```python
from build123d import *

# Parameters (mm, degrees)
SKETCH_2_R      = 300
SKETCH_2_R_2    = 3
EXTRUDE_1_DEPTH = 20


with BuildPart() as part:
    # Эскиз2 → Бобышка-Вытянуть1 (new body)
    with BuildSketch(Plane(origin=(0, 0, 0), x_dir=(1, 0, 0), z_dir=(0, 1, 0))):
        with Locations(Location((0, 0, 0), (0, 0, 270))):
            Circle(SKETCH_2_R)
        with Locations(Location((-50, 50, 0), (0, 0, 270))):
            Circle(SKETCH_2_R_2, mode=Mode.SUBTRACT)
        with Locations(Location((-100, 50, 0), (0, 0, 270))):
            Circle(SKETCH_2_R_2, mode=Mode.SUBTRACT)
        with Locations(Location((-150, 50, 0), (0, 0, 270))):
            Circle(SKETCH_2_R_2, mode=Mode.SUBTRACT)
        with Locations(Location((-200, 50, 0), (0, 0, 270))):
            Circle(SKETCH_2_R_2, mode=Mode.SUBTRACT)
        with Locations(Location((-50, 100, 0), (0, 0, 270))):
            Circle(SKETCH_2_R_2, mode=Mode.SUBTRACT)
        with Locations(Location((-100, 100, 0), (0, 0, 270))):
            Circle(SKETCH_2_R_2, mode=Mode.SUBTRACT)
        with Locations(Location((-150, 100, 0), (0, 0, 270))):
            Circle(SKETCH_2_R_2, mode=Mode.SUBTRACT)
        with Locations(Location((-200, 100, 0), (0, 0, 270))):
            Circle(SKETCH_2_R_2, mode=Mode.SUBTRACT)
        with Locations(Location((-250, 100, 0), (0, 0, 270))):
            Circle(SKETCH_2_R_2, mode=Mode.SUBTRACT)
        with Locations(Location((-50, 150, 0), (0, 0, 270))):
            Circle(SKETCH_2_R_2, mode=Mode.SUBTRACT)
        with Locations(Location((-100, 150, 0), (0, 0, 270))):
            Circle(SKETCH_2_R_2, mode=Mode.SUBTRACT)
        with Locations(Location((-150, 150, 0), (0, 0, 270))):
            Circle(SKETCH_2_R_2, mode=Mode.SUBTRACT)
        with Locations(Location((-200, 150, 0), (0, 0, 270))):
            Circle(SKETCH_2_R_2, mode=Mode.SUBTRACT)
        with Locations(Location((-50, 200, 0), (0, 0, 270))):
            Circle(SKETCH_2_R_2, mode=Mode.SUBTRACT)
        with Locations(Location((-100, 200, 0), (0, 0, 270))):
            Circle(SKETCH_2_R_2, mode=Mode.SUBTRACT)
        with Locations(Location((-150, 200, 0), (0, 0, 270))):
            Circle(SKETCH_2_R_2, mode=Mode.SUBTRACT)
        with Locations(Location((-100, 250, 0), (0, 0, 270))):
            Circle(SKETCH_2_R_2, mode=Mode.SUBTRACT)
        with Locations(Location((-50, 0, 0), (0, 0, 270))):
            Circle(SKETCH_2_R_2, mode=Mode.SUBTRACT)
        with Locations(Location((-150, 0, 0), (0, 0, 270))):
            Circle(SKETCH_2_R_2, mode=Mode.SUBTRACT)
        with Locations(Location((-100, 0, 0), (0, 0, 270))):
            Circle(SKETCH_2_R_2, mode=Mode.SUBTRACT)
        with Locations(Location((-200, 0, 0), (0, 0, 270))):
            Circle(SKETCH_2_R_2, mode=Mode.SUBTRACT)
        with Locations(Location((0, 50, 0), (0, 0, 270))):
            Circle(SKETCH_2_R_2, mode=Mode.SUBTRACT)
        with Locations(Location((0, 100, 0), (0, 0, 270))):
            Circle(SKETCH_2_R_2, mode=Mode.SUBTRACT)
        with Locations(Location((0, 150, 0), (0, 0, 270))):
            Circle(SKETCH_2_R_2, mode=Mode.SUBTRACT)
        with Locations(Location((0, 200, 0), (0, 0, 270))):
            Circle(SKETCH_2_R_2, mode=Mode.SUBTRACT)
        with Locations(Location((200, 0, 0), (0, 0, 90))):
            Circle(SKETCH_2_R_2, mode=Mode.SUBTRACT)
        with Locations(Location((100, 0, 0), (0, 0, 90))):
            Circle(SKETCH_2_R_2, mode=Mode.SUBTRACT)
        with Locations(Location((150, 0, 0), (0, 0, 90))):
            Circle(SKETCH_2_R_2, mode=Mode.SUBTRACT)
        with Locations(Location((50, 0, 0), (0, 0, 90))):
            Circle(SKETCH_2_R_2, mode=Mode.SUBTRACT)
        with Locations(Location((100, 250, 0), (0, 0, 90))):
            Circle(SKETCH_2_R_2, mode=Mode.SUBTRACT)
        with Locations(Location((150, 200, 0), (0, 0, 90))):
            Circle(SKETCH_2_R_2, mode=Mode.SUBTRACT)
        with Locations(Location((100, 200, 0), (0, 0, 90))):
            Circle(SKETCH_2_R_2, mode=Mode.SUBTRACT)
        with Locations(Location((50, 200, 0), (0, 0, 90))):
            Circle(SKETCH_2_R_2, mode=Mode.SUBTRACT)
        with Locations(Location((200, 150, 0), (0, 0, 90))):
            Circle(SKETCH_2_R_2, mode=Mode.SUBTRACT)
        with Locations(Location((150, 150, 0), (0, 0, 90))):
            Circle(SKETCH_2_R_2, mode=Mode.SUBTRACT)
        with Locations(Location((100, 150, 0), (0, 0, 90))):
            Circle(SKETCH_2_R_2, mode=Mode.SUBTRACT)
        with Locations(Location((50, 150, 0), (0, 0, 90))):
            Circle(SKETCH_2_R_2, mode=Mode.SUBTRACT)
        with Locations(Location((250, 100, 0), (0, 0, 90))):
            Circle(SKETCH_2_R_2, mode=Mode.SUBTRACT)
        with Locations(Location((200, 100, 0), (0, 0, 90))):
            Circle(SKETCH_2_R_2, mode=Mode.SUBTRACT)
        with Locations(Location((150, 100, 0), (0, 0, 90))):
            Circle(SKETCH_2_R_2, mode=Mode.SUBTRACT)
        with Locations(Location((100, 100, 0), (0, 0, 90))):
            Circle(SKETCH_2_R_2, mode=Mode.SUBTRACT)
        with Locations(Location((50, 100, 0), (0, 0, 90))):
            Circle(SKETCH_2_R_2, mode=Mode.SUBTRACT)
        with Locations(Location((200, 50, 0), (0, 0, 90))):
            Circle(SKETCH_2_R_2, mode=Mode.SUBTRACT)
        with Locations(Location((150, 50, 0), (0, 0, 90))):
            Circle(SKETCH_2_R_2, mode=Mode.SUBTRACT)
        with Locations(Location((100, 50, 0), (0, 0, 90))):
            Circle(SKETCH_2_R_2, mode=Mode.SUBTRACT)
        with Locations(Location((50, 50, 0), (0, 0, 90))):
            Circle(SKETCH_2_R_2, mode=Mode.SUBTRACT)
        with Locations(Location((50, -50, 0), (0, 0, 270))):
            Circle(SKETCH_2_R_2, mode=Mode.SUBTRACT)
        with Locations(Location((100, -50, 0), (0, 0, 270))):
            Circle(SKETCH_2_R_2, mode=Mode.SUBTRACT)
        with Locations(Location((150, -50, 0), (0, 0, 270))):
            Circle(SKETCH_2_R_2, mode=Mode.SUBTRACT)
        with Locations(Location((200, -50, 0), (0, 0, 270))):
            Circle(SKETCH_2_R_2, mode=Mode.SUBTRACT)
        with Locations(Location((50, -100, 0), (0, 0, 270))):
            Circle(SKETCH_2_R_2, mode=Mode.SUBTRACT)
        with Locations(Location((100, -100, 0), (0, 0, 270))):
            Circle(SKETCH_2_R_2, mode=Mode.SUBTRACT)
        with Locations(Location((150, -100, 0), (0, 0, 270))):
            Circle(SKETCH_2_R_2, mode=Mode.SUBTRACT)
        with Locations(Location((200, -100, 0), (0, 0, 270))):
            Circle(SKETCH_2_R_2, mode=Mode.SUBTRACT)
        with Locations(Location((250, -100, 0), (0, 0, 270))):
            Circle(SKETCH_2_R_2, mode=Mode.SUBTRACT)
        with Locations(Location((50, -150, 0), (0, 0, 270))):
            Circle(SKETCH_2_R_2, mode=Mode.SUBTRACT)
        with Locations(Location((100, -150, 0), (0, 0, 270))):
            Circle(SKETCH_2_R_2, mode=Mode.SUBTRACT)
        with Locations(Location((150, -150, 0), (0, 0, 270))):
            Circle(SKETCH_2_R_2, mode=Mode.SUBTRACT)
        with Locations(Location((200, -150, 0), (0, 0, 270))):
            Circle(SKETCH_2_R_2, mode=Mode.SUBTRACT)
        with Locations(Location((50, -200, 0), (0, 0, 270))):
            Circle(SKETCH_2_R_2, mode=Mode.SUBTRACT)
        with Locations(Location((100, -200, 0), (0, 0, 270))):
            Circle(SKETCH_2_R_2, mode=Mode.SUBTRACT)
        with Locations(Location((150, -200, 0), (0, 0, 270))):
            Circle(SKETCH_2_R_2, mode=Mode.SUBTRACT)
        with Locations(Location((100, -250, 0), (0, 0, 270))):
            Circle(SKETCH_2_R_2, mode=Mode.SUBTRACT)
        with Locations(Location((0, -200, 0), (0, 0, 90))):
            Circle(SKETCH_2_R_2, mode=Mode.SUBTRACT)
        with Locations(Location((0, -150, 0), (0, 0, 90))):
            Circle(SKETCH_2_R_2, mode=Mode.SUBTRACT)
        with Locations(Location((0, -100, 0), (0, 0, 90))):
            Circle(SKETCH_2_R_2, mode=Mode.SUBTRACT)
        with Locations(Location((0, -50, 0), (0, 0, 90))):
            Circle(SKETCH_2_R_2, mode=Mode.SUBTRACT)
        with Locations(Location((-100, -250, 0), (0, 0, 90))):
            Circle(SKETCH_2_R_2, mode=Mode.SUBTRACT)
        with Locations(Location((-150, -200, 0), (0, 0, 90))):
            Circle(SKETCH_2_R_2, mode=Mode.SUBTRACT)
        with Locations(Location((-100, -200, 0), (0, 0, 90))):
            Circle(SKETCH_2_R_2, mode=Mode.SUBTRACT)
        with Locations(Location((-50, -200, 0), (0, 0, 90))):
            Circle(SKETCH_2_R_2, mode=Mode.SUBTRACT)
        with Locations(Location((-200, -150, 0), (0, 0, 90))):
            Circle(SKETCH_2_R_2, mode=Mode.SUBTRACT)
        with Locations(Location((-150, -150, 0), (0, 0, 90))):
            Circle(SKETCH_2_R_2, mode=Mode.SUBTRACT)
        with Locations(Location((-100, -150, 0), (0, 0, 90))):
            Circle(SKETCH_2_R_2, mode=Mode.SUBTRACT)
        with Locations(Location((-50, -150, 0), (0, 0, 90))):
            Circle(SKETCH_2_R_2, mode=Mode.SUBTRACT)
        with Locations(Location((-250, -100, 0), (0, 0, 90))):
            Circle(SKETCH_2_R_2, mode=Mode.SUBTRACT)
        with Locations(Location((-200, -100, 0), (0, 0, 90))):
            Circle(SKETCH_2_R_2, mode=Mode.SUBTRACT)
        with Locations(Location((-150, -100, 0), (0, 0, 90))):
            Circle(SKETCH_2_R_2, mode=Mode.SUBTRACT)
        with Locations(Location((-100, -100, 0), (0, 0, 90))):
            Circle(SKETCH_2_R_2, mode=Mode.SUBTRACT)
        with Locations(Location((-50, -100, 0), (0, 0, 90))):
            Circle(SKETCH_2_R_2, mode=Mode.SUBTRACT)
        with Locations(Location((-200, -50, 0), (0, 0, 90))):
            Circle(SKETCH_2_R_2, mode=Mode.SUBTRACT)
        with Locations(Location((-150, -50, 0), (0, 0, 90))):
            Circle(SKETCH_2_R_2, mode=Mode.SUBTRACT)
        with Locations(Location((-100, -50, 0), (0, 0, 90))):
            Circle(SKETCH_2_R_2, mode=Mode.SUBTRACT)
        with Locations(Location((-50, -50, 0), (0, 0, 90))):
            Circle(SKETCH_2_R_2, mode=Mode.SUBTRACT)
    extrude(amount=EXTRUDE_1_DEPTH)


solid = part.part
```
Part model, mm, in its own coordinate system. Round coordinates to 2 decimals unless told otherwise and drop trailing zeros. Write each loop counter-clockwise with the first axis right and the second up, starting at its lowest first coordinate (ties: lowest second). Pieces come first, ordered by that corner, then holes. Notation, with made-up numbers: M -12,-2 L 25,-2 A21 cw 25,33 Z; hole C 3.25,22.25 d10. An arc over 180 degrees is marked long. One line per question, with ' | ' between items.
(1) Saw through at A-A on y = 13. Count the separate pieces of the cut face and the enclosed holes in it, then the cut area to 3 significant figures.
Answer key:
separate pieces: 1 | enclosed holes: 84 | area: 280,000 mm^2
(2) Probe line 1 along X through (y, z) = (15.25, 260.5); line 2 along X through (y, z) = (3, -155); line 3 along Z through (x, y) = (132, 15.25). List the from-to ranges inside material, lowest first.
Answer key:
line 1: x = -148.79 to 148.79 | line 2: x = -256.86 to 256.86 | line 3: z = -269.4 to 269.4
(3) Pin check, flat tips, straight feed: pin 1 (2 mm diameter, centred on x = -106, y = 14.5, fed in from -Z); pin 2 (12 mm diameter, centred on y = 12, z = -97, fed in from -X); pin 3 (8 mm diameter, centred on x = 108.5, y = 16, fed in from +Z). Stop position of each tip, or through.
Answer key:
pin 1: stops at z = -281.02 | pin 2: stops at x = -285.87 | pin 3: stops at z = 281.21
(4) Saw through at C-C on z = 135. Write the cut outline in (x, y).
Answer key:
outline: M -267.91,0 L 267.91,0 L 267.91,20 L -267.91,20 Z
(5) Saw through at B-B on x = -76. Write the cut outline in (y, z).
Answer key:
outline: M 0,-290.21 L 20,-290.21 L 20,290.21 L 0,290.21 Z
